Study the drawing (mm; zero at the part's minimum x, y, z) and answer. Coordinates: 2 decimals unless noted, no trailing zeros. Order: outer loops, then holes, each group sorted by start corner. A loop starts at its lowest first (then second) coordinate and runs counter-clockwise, first axis right, second up. Notation, with made-up numbers: (-8.75, -9) -> (-1.75, -9) arc R22 cw to (-1.75, 26) -> close; hole circle Ø10 at (9, 73). An arc over 180 degrees is marked (long way). Answer as CSV lines item,"result". Start each with the question number.
Item 1: Section B-B (z = 7.75) is taken. Write down the section's boundary in (x, y) (1 decimal), then the cut area to 3 significant figures.
Item 2: Section D-D (z = 3) is taken. Write down the section's boundary in (x, y) (1 decimal).
Item 3: Section C-C (x = 1.2) is taken. Count the separate pieces of the cut face and the enclosed holes in it, then the cut area to 3 significant figures.
Item 4: Section A-A (y = 20) is taken. Write down the section's boundary in (x, z) (1 decimal).
Item 5: Straight lines are drawn through the part: L1, parallel to Y at x = 4.55, z = 14.5 (1 decimal); L2, parallel to Y at x = 4.75, z = 5.5 (1 decimal); L3, parallel to Y at x = 0.45, z = 12. For each, find the intervals that lie inside material, in ascending order.
Item 6: Each of these flat-tipped pins is pushed along its axis until it touches: pin 1 Ø1 at (x, z) = (3, 10.5) entering from +Y; pin 2 Ø1 at (x, z) = (2.5, 10.5) entering from -Y. Where does it stop, or does it pass through?
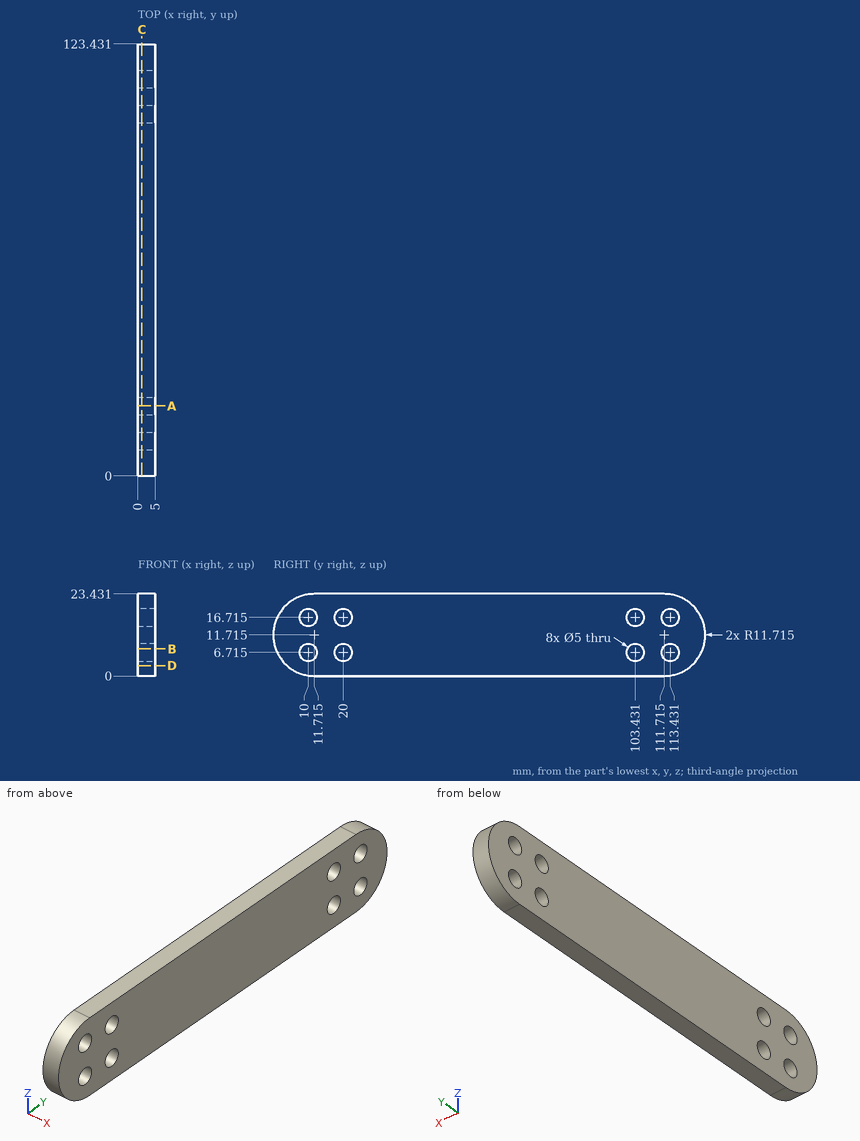
Checked values:
1,outline,"(0, 0.7) -> (5, 0.7) -> (5, 7.7) -> (0, 7.7) -> close; (0, 12.3) -> (5, 12.3) -> (5, 17.7) -> (0, 17.7) -> close; (0, 22.3) -> (5, 22.3) -> (5, 101.2) -> (0, 101.2) -> close; (0, 105.7) -> (5, 105.7) -> (5, 111.2) -> (0, 111.2) -> close; (0, 115.7) -> (5, 115.7) -> (5, 122.7) -> (0, 122.7) -> close"
1,area,"519 mm^2"
2,outline,"(0, 3.9) -> (5, 3.9) -> (5, 119.5) -> (0, 119.5) -> close"
3,separate pieces,"1"
3,enclosed holes,"8"
3,area,"2,620 mm^2"
4,outline,"(0, 0) -> (5, 0) -> (5, 4.2) -> (0, 4.2) -> close; (0, 9.2) -> (5, 9.2) -> (5, 14.2) -> (0, 14.2) -> close; (0, 19.2) -> (5, 19.2) -> (5, 23.4) -> (0, 23.4) -> close"
5,L1,"y = 0.3 to 8.8, 11.2 to 18.8, 21.2 to 102.3, 104.6 to 112.3, 114.6 to 123.1"
5,L2,"y = 1.8 to 7.8, 12.2 to 17.8, 22.2 to 101.2, 105.6 to 111.2, 115.6 to 121.6"
5,L3,"y = 0 to 123.43"
6,pin 1,"stops at y = 123.41"
6,pin 2,"stops at y = 0.02"
